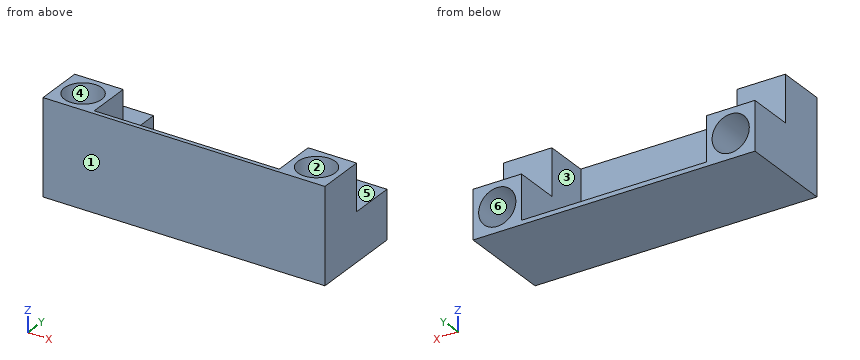
```python
from build123d import *

# Parameters (mm, degrees)
SKETCH1_R           = 13.2
BOSS_EXTRUDE3_DEPTH = 5
SKETCH1_6_W         = 100
SKETCH1_6_H         = 55
SKETCH1_6_R         = 13.2
BOSS_EXTRUDE4_DEPTH = 55
SKETCH2_W           = 65.6
SKETCH2_H           = 52
CUT_EXTRUDE1_DEPTH  = 52
SKETCH3_R           = 13.2
CUT_EXTRUDE2_DEPTH  = 22.6
SKETCH4_W           = 20.6
SKETCH4_H           = 20.6
CUT_EXTRUDE4_DEPTH  = 39
SKETCH9_R           = 13.2
BOSS_EXTRUDE5_DEPTH = 12.4
BOSS_EXTRUDE7_START = 12.4
SKETCH10_R          = 13.2
BOSS_EXTRUDE7_DEPTH = 12.4
MIRROR1_START       = 30.398461356
MIRROR1_OUTLINE_R   = 13.2
MIRROR1_DEPTH       = 37.001538644
MIRROR1_2_OUTLINE_W = 100
MIRROR1_2_OUTLINE_H = 67.4
MIRROR1_2_OUTLINE_R = 13.2
MIRROR1_2_DEPTH     = 3
MIRROR1_3_OUTLINE_W = 34.4
MIRROR1_3_OUTLINE_H = 33
MIRROR1_3_DEPTH     = 4.001538644
MIRROR1_START_2     = 3
MIRROR1_4_OUTLINE_R = 13.2
MIRROR1_4_DEPTH     = 0.998461256
MIRROR1_START_3     = 3.998461256
MIRROR1_5_OUTLINE_R = 13.2
MIRROR1_5_DEPTH     = 26.4000001
MIRROR1_START_4     = 4.9
MIRROR1_6_OUTLINE_R = 13.2
MIRROR1_6_DEPTH     = 35


with BuildPart() as part:
    # Sketch1 → Boss-Extrude3 (new body)
    with BuildSketch(Plane(origin=(0, 0, 0), x_dir=(1, 0, 0), z_dir=(0, 1, 0))):
        with Locations(Location((-32.8, 10.3, 0), (0, 0, 270))):
            Circle(SKETCH1_R)
    boss_extrude3 = extrude(amount=BOSS_EXTRUDE3_DEPTH)

    # Sketch1<6> → Boss-Extrude4 (add)
    with BuildSketch(Plane(origin=(0, 0, 0), x_dir=(1, 0, 0), z_dir=(0, 1, 0))):
        Rectangle(SKETCH1_6_W, SKETCH1_6_H)
        with Locations(Location((-32.8, 10.3, 0), (0, 0, 270))):
            Circle(SKETCH1_6_R, mode=Mode.SUBTRACT)
    extrude(amount=BOSS_EXTRUDE4_DEPTH)

    # Sketch2 → Cut-Extrude1 (cut)
    with BuildSketch(Plane(origin=(0, 55, 0), x_dir=(1, 0, 0), z_dir=(0, 1, 0))):
        with Locations((17.2, -1.5)):
            Rectangle(SKETCH2_W, SKETCH2_H)
    extrude(amount=-CUT_EXTRUDE1_DEPTH, mode=Mode.SUBTRACT)

    # Sketch3 → Cut-Extrude2 (cut)
    with BuildSketch(Plane.XY.offset(27.5)):
        with Locations((-32.801538644, 17.198461356)):
            Circle(SKETCH3_R)
    extrude(amount=-CUT_EXTRUDE2_DEPTH, mode=Mode.SUBTRACT)

    # Sketch4 → Cut-Extrude4 (cut)
    with BuildSketch(Plane.ZY.offset(50)):
        with Locations((17.2, 44.7)):
            Rectangle(SKETCH4_W, SKETCH4_H)
    extrude(amount=-CUT_EXTRUDE4_DEPTH, mode=Mode.SUBTRACT)

    # Sketch9 → Boss-Extrude5 (add)
    with BuildSketch(Plane(origin=(0, 55, 0), x_dir=(1, 0, 0), z_dir=(0, 1, 0))):
        Polygon((-50, -6.9), (-15.6, -6.9), (-15.6, 24.5), (50, 24.5), (50, 27.5), (-50, 27.5), align=None)
        with Locations(Location((-32.8, 10.3, 0), (0, 0, 270))):
            Circle(SKETCH9_R, mode=Mode.SUBTRACT)
    extrude(amount=BOSS_EXTRUDE5_DEPTH)

    # Sketch10 → Boss-Extrude7 (add)
    with BuildSketch(Plane.XY.offset(27.5).offset(BOSS_EXTRUDE7_START)):
        Polygon((-15.6, 3), (-15.6, 34.4), (-50, 34.4), (-50, 0), (50, 0), (50, 3), align=None)
        with Locations((-32.801538644, 17.198461356)):
            Circle(SKETCH10_R, mode=Mode.SUBTRACT)
    extrude(amount=-BOSS_EXTRUDE7_DEPTH)

    # Mirror1: read off the stored shape, not the designer's step
    # Mirror1 outline → Mirror1 (add)
    with BuildSketch(Plane(origin=(0, 0, 0), x_dir=(1, 0, 0), z_dir=(0, 1, 0)).offset(MIRROR1_START)):
        Polygon((150, -6.9), (150, 27.5), (50, 27.5), (50, 24.5), (115.6, 24.5), (115.6, -6.9), align=None)
        with Locations((132.8, 10.3)):
            Circle(MIRROR1_OUTLINE_R, mode=Mode.SUBTRACT)
    extrude(amount=MIRROR1_DEPTH)

    # Mirror1 2 outline → Mirror1 2 (add)
    with BuildSketch(Plane(origin=(0, 0, 0), x_dir=(1, 0, 0), z_dir=(0, 1, 0))):
        with Locations((100, -6.2)):
            Rectangle(MIRROR1_2_OUTLINE_W, MIRROR1_2_OUTLINE_H)
        with Locations((132.8, 10.3)):
            Circle(MIRROR1_2_OUTLINE_R, mode=Mode.SUBTRACT)
    extrude(amount=MIRROR1_2_DEPTH)

    # Mirror1 3 outline → Mirror1 3 (add)
    with BuildSketch(Plane(origin=(0, 0, 0), x_dir=(1, 0, 0), z_dir=(0, 1, 0)).offset(MIRROR1_START)):
        with Locations((132.8, -23.4)):
            Rectangle(MIRROR1_3_OUTLINE_W, MIRROR1_3_OUTLINE_H)
    extrude(amount=MIRROR1_3_DEPTH)

    # Mirror1 4 outline → Mirror1 4 (add)
    with BuildSketch(Plane(origin=(0, 0, 0), x_dir=(1, 0, 0), z_dir=(0, 1, 0)).offset(MIRROR1_START_2)):
        Polygon((150, 27.5), (50, 27.5), (50, 24.5), (115.6, 24.5), (115.6, -39.9), (150, -39.9), align=None)
        with Locations((132.8, 10.3)):
            Circle(MIRROR1_4_OUTLINE_R, mode=Mode.SUBTRACT)
    extrude(amount=MIRROR1_4_DEPTH)

    # Mirror1 5 outline → Mirror1 5 (add)
    with BuildSketch(Plane(origin=(0, 0, 0), x_dir=(1, 0, 0), z_dir=(0, 1, 0)).offset(MIRROR1_START_3)):
        Polygon((150, -39.9), (150, 27.5), (50, 27.5), (50, 24.5), (115.6, 24.5), (115.6, -39.9), align=None)
        with Locations((132.8, 10.3)):
            Circle(MIRROR1_5_OUTLINE_R, mode=Mode.SUBTRACT)
    extrude(amount=MIRROR1_5_DEPTH)

    # Mirror1 6 outline → Mirror1 6 (cut)
    with BuildSketch(Plane.XY.offset(MIRROR1_START_4)):
        with Locations((132.801538644, 17.198461356)):
            Circle(MIRROR1_6_OUTLINE_R)
    extrude(amount=MIRROR1_6_DEPTH, mode=Mode.SUBTRACT)

    # Mirror2: Boss-Extrude3 across plane
    add(boss_extrude3.mirror(Plane.ZY.offset(-50)))


solid = part.part
```
Source: CAD feature listing. Evaluate the final solid. Frame: model axes, mm. Face numbers are marked on the shaded views. A direction names the side the tool comes from. Coordinates: 2 decimals unless noted, no trailing zeros. Write each loop counter-clockwise with the first axis right and the second up, starting at its lowest first coordinate (ties: lowest second). Pieces come first, ordered by that corner, then holes. Notation, with made-up numbers: (66.25, -38.75) -> (80.25, -38.75) arc R25 ccw to (80.25, -7.75) -> close; hole circle Ø4 at (-4, 53). An arc over 180 degrees is marked (long way). Return JSON: item names as keys, results as strings. Group by question number.
1) Section query B-B, the plane x = 132.8. Return loops of the section in (y, z).
2) Contact query for flat-ended pins moving along their axis: P1, Ø8, axis at x = 133.5, y = 12.5, coming from the +Z side; P2, Ø8, axis at x = -12.5, z = 3, coming from the +Y side; P3, Ø24, axis at x = -32.8, z = -10.3, coming from the +Y side; P4, Ø16.5, axis at x = 131.5, y = 54.5, coming from the +Z side. Output: stop coordinate, or through.
3) Set-up query: the marked faces 4, 5 and 6. Return all of +Z, -Z, +X, -X, +Y, -Y with unobstructed straight access to the full face (end or side cutting, diameter ignored); none if empty.
4) Section query A-A, the plane y = 51. Return loops of the section in (x, z).
5) Mould query, pull axis Y, two halves, no side actions, for the marked faces 1, 2 and 3. Classes: +Y half, -Y half, draft (parallel to the pull), parting line (faces both ways), or undercut.
6) Section query C-C, the plane z = -10.3. Return loops of the section in (x, y).
7) Section query D-D, the plane z = 18. Return loops of the section in (x, y), plus the area to 3 significant figures.
8) Ray query, line 1 along X through (y, z) = (46, -10); line 2 along X through (y, z) = (57, -3.5); line 3 along Z through (x, y) = (-32, 55). Return the intervals inside material, ascending.
From the geometry:
{
 "1": {"outline": "(0, -27.5) -> (67.4, -27.5) -> (67.4, -23.5) -> (5, -23.5) -> (5, 2.9) -> (67.4, 2.9) -> (67.4, 6.9) -> (34.4, 6.9) -> (34.4, 39.9) -> (30.4, 39.9) -> (30.4, 4.9) -> (4, 4.9) -> (4, 39.9) -> (0, 39.9) -> close"},
 "2": {"P1": "z = 4.9", "P2": "y = 67.4", "P3": "y = 5", "P4": "z = 6.9"},
 "3": {"face 4": "+Z", "face 5": "+Z, +X, -X, +Y", "face 6": "+Y"},
 "4": {"outline": "(-50, -27.5) -> (150, -27.5) -> (150, 6.9) -> (115.6, 6.9) -> (115.6, -24.5) -> (-15.6, -24.5) -> (-15.6, 6.9) -> (-50, 6.9) -> close; hole circle Ø26.4 at (-32.8, -10.3); hole circle Ø26.4 at (132.8, -10.3)"},
 "5": {"face 1": "-Y half", "face 2": "undercut", "face 3": "draft"},
 "6": {"outline": "(-50, 0) -> (150, 0) -> (150, 67.4) -> (146, 67.4) -> (146, 5) -> (119.6, 5) -> (119.6, 67.4) -> (115.6, 67.4) -> (115.6, 3) -> (-15.6, 3) -> (-15.6, 67.4) -> (-19.6, 67.4) -> (-19.6, 5) -> (-46, 5) -> (-46, 67.4) -> (-50, 67.4) -> close"},
 "7": {"outline": "(-50, 0) -> (150, 0) -> (150, 34.4) -> (115.6, 34.4) -> (115.6, 3) -> (-15.6, 3) -> (-15.6, 34.4) -> (-50, 34.4) -> close; hole circle Ø26.4 at (-32.8, 17.2); hole circle Ø26.4 at (132.8, 17.2)", "area": "1,670 mm²"},
 "8": {"line 1": "-50 to -46, -19.6 to -15.6, 115.6 to 119.6, 146 to 150", "line 2": "-50 to -44.11, -21.49 to -15.6, 115.6 to 121.49, 144.11 to 150", "line 3": "-27.5 to -23.48, 2.88 to 6.9"}
}
